For this review, take the finished solid that the model builds, in its own axes (mm). Give positions to 0.01 mm unless a question says otherwise; leave off trailing zeros. Write each loop counter-clockwise with the first axis right and the second up, starting at its lowest first coordinate (ties: lowest second). Pieces come first, ordered by that corner, then holes. Notation, with made-up numbers: M -5,23 L 17,23 A5 cw 17,31 Z; hole C -3.5,-29 d5. An arc over 180 degrees is marked long. One line per item, written item: value. Start each with the question number.
Item 1: Consider section B-B, the plane y = 1.2. Give the number of separate pieces and of enclosed holes in the cut face, and give its area (3 significant figures).
Item 2: Clearance check with flat-ended pins moving along their axes: pin 1 Ø3.5 at (x, z) = (70.83, -255.23) entering from +Y; pin 2 Ø10 at (x, z) = (48.5, -149) entering from -Y; pin 3 Ø1.6 at (y, z) = (1, -276) entering from -X (3 decimals). State where each tip first meets the part, or that it passes through.
Item 3: Consider section A-A, the plane z = -286. Write out the cut boundary in (x, y) (3 decimals), and give its area (3 significant figures).
Item 4: To check wall thickness, follow probe 1 along Z at (x, y) = (191.77, 0.9) (1 decimal); probe 2 along X at (y, z) = (1.3, 6.35); probe 3 along Z at (x, y) = (26, 0.2) (3 decimals). State the ranges of each line that lie inside material, in increasing order.
```python
from build123d import *

# Parameters (mm, degrees)
SKETCH1_W           = 210.82
SKETCH1_H           = 257.175
SKETCH1_W_2         = 185.42
SKETCH1_H_2         = 231.775
BOSS_EXTRUDE1_DEPTH = 3.175
SKETCH3_R           = 2.0955
CUT_EXTRUDE1_DEPTH  = 3.175
SKETCH3_3_R         = 45.33
SKETCH3_3_W         = 107.95
SKETCH3_3_H         = 21.4884
BOSS_EXTRUDE2_DEPTH = 3.175
FILLET1_R           = 2.54
SKETCH4_R           = 2.0955
CUT_EXTRUDE2_DEPTH  = 3.175


with BuildPart() as part:
    # Sketch1 → Boss-Extrude1 (new body)
    with BuildSketch(Plane(origin=(0, 0, 0), x_dir=(1, 0, 0), z_dir=(0, 1, 0))):
        with Locations((92.71, 115.8875)):
            Rectangle(SKETCH1_W, SKETCH1_H)
        with Locations((92.71, 115.8875)):
            Rectangle(SKETCH1_W_2, SKETCH1_H_2, mode=Mode.SUBTRACT)
        with Locations((92.71, 115.8875)):
            Rectangle(SKETCH1_W_2, SKETCH1_H_2)
    extrude(amount=BOSS_EXTRUDE1_DEPTH)

    # Sketch3 → Cut-Extrude1 (cut)
    with BuildSketch(Plane(origin=(0, 3.175, 0), x_dir=(1, 0, 0), z_dir=(0, 1, 0))):
        with Locations(Location((191.77, 238.125, 0), (0, 0, 270))):
            Circle(SKETCH3_R)
        with Locations(Location((191.77, -6.35, 0), (0, 0, 270))):
            Circle(SKETCH3_R)
        with Locations(Location((-6.35, -6.35, 0), (0, 0, 270))):
            Circle(SKETCH3_R)
        with Locations(Location((-6.35, 238.125, 0), (0, 0, 270))):
            Circle(SKETCH3_R)
    extrude(amount=-CUT_EXTRUDE1_DEPTH, mode=Mode.SUBTRACT)

    # Sketch3<3> → Boss-Extrude2 (add)
    with BuildSketch(Plane(origin=(0, 3.175, 0), x_dir=(1, 0, 0), z_dir=(0, 1, 0))):
        with BuildLine():
            ThreePointArc((138.04, 277.105), (134.430200877, 259.378360759), (124.175727387, 244.475))
            Line((124.175727387, 244.475), (146.685, 244.475))
            Line((146.685, 244.475), (146.685, 301.625))
            Line((146.685, 301.625), (142.4305, 301.625))
            ThreePointArc((142.4305, 301.625), (138.85325774, 300.14325774), (140.335, 303.7205))
            Line((140.335, 303.7205), (140.335, 307.975))
            Line((140.335, 307.975), (125.904156112, 307.975))
            ThreePointArc((125.904156112, 307.975), (134.897083311, 293.68989981), (138.04, 277.105))
        make_face()
        with BuildLine():
            Line((142.4305, 301.625), (146.685, 301.625))
            Line((146.685, 301.625), (146.685, 307.975))
            Line((146.685, 307.975), (140.335, 307.975))
            Line((140.335, 307.975), (140.335, 303.7205))
            ThreePointArc((140.335, 303.7205), (141.81674226, 303.10674226), (142.4305, 301.625))
        make_face()
        with BuildLine():
            Line((38.735, 244.475), (61.244272613, 244.475))
            ThreePointArc((61.244272613, 244.475), (47.396783015, 275.871603687), (59.515843888, 307.975))
            Line((59.515843888, 307.975), (45.085, 307.975))
            Line((45.085, 307.975), (45.085, 303.7205))
            ThreePointArc((45.085, 303.7205), (46.56674226, 303.10674226), (47.1805, 301.625))
            ThreePointArc((47.1805, 301.625), (45.085, 299.5295), (42.9895, 301.625))
            Line((42.9895, 301.625), (38.735, 301.625))
            Line((38.735, 301.625), (38.735, 244.475))
        make_face()
        with BuildLine():
            Line((38.735, 307.975), (38.735, 301.625))
            Line((38.735, 301.625), (42.9895, 301.625))
            ThreePointArc((42.9895, 301.625), (43.60325774, 303.10674226), (45.085, 303.7205))
            Line((45.085, 303.7205), (45.085, 307.975))
            Line((45.085, 307.975), (38.735, 307.975))
        make_face()
        with BuildLine():
            ThreePointArc((61.244272613, 244.475), (75.743989862, 235.069736233), (92.71, 231.775))
            Line((92.71, 231.775), (92.71, 244.475))
            Line((92.71, 244.475), (61.244272613, 244.475))
        make_face()
        with BuildLine():
            Line((92.71, 244.475), (92.71, 231.775))
            ThreePointArc((92.71, 231.775), (109.676010138, 235.069736233), (124.175727387, 244.475))
            Line((124.175727387, 244.475), (92.71, 244.475))
        make_face()
        with Locations((92.71, 277.105)):
            Circle(SKETCH3_3_R)
        with Locations((92.71, 318.7192)):
            Rectangle(SKETCH3_3_W, SKETCH3_3_H)
        with BuildLine():
            Line((59.515843888, 307.975), (92.71, 307.975))
            Line((92.71, 307.975), (92.71, 322.435))
            ThreePointArc((92.71, 322.435), (74.606522434, 318.663067809), (59.515843888, 307.975))
        make_face()
        with BuildLine():
            Line((92.71, 322.435), (92.71, 307.975))
            Line((92.71, 307.975), (125.904156112, 307.975))
            ThreePointArc((125.904156112, 307.975), (110.813477566, 318.663067809), (92.71, 322.435))
        make_face()
    extrude(amount=-BOSS_EXTRUDE2_DEPTH)

    # Fillet1
    fillet1_edges = [part.edges().sort_by_distance(p)[0] for p in [
        (146.685, 1.5875, -244.475),
        (38.735, 1.5875, -244.475),
        (38.735, 1.5875, -329.4634),
        (146.685, 1.5875, -329.4634),
        (-12.7, 1.5875, -244.475),
        (198.12, 1.5875, -244.475),
        (198.12, 1.5875, 12.7),
        (-12.7, 1.5875, 12.7),
    ]]
    fillet(fillet1_edges, radius=FILLET1_R)

    # Sketch4 → Cut-Extrude2 (cut)
    with BuildSketch(Plane(origin=(0, 3.175, 0), x_dir=(1, 0, 0), z_dir=(0, 1, 0))):
        with Locations(Location((70.834096089, 298.980903911, 0), (0, 0, 270))):
            Circle(SKETCH4_R)
        with Locations(Location((114.585903911, 298.980903911, 0), (0, 0, 270))):
            Circle(SKETCH4_R)
        with Locations(Location((114.585903911, 255.229096089, 0), (0, 0, 270))):
            Circle(SKETCH4_R)
        with Locations(Location((70.834096089, 255.229096089, 0), (0, 0, 270))):
            Circle(SKETCH4_R)
    extrude(amount=-CUT_EXTRUDE2_DEPTH, mode=Mode.SUBTRACT)


solid = part.part
```
Model answer:
1. separate pieces: 1
1. enclosed holes: 10
1. area: 63,200 mm2
2. pin 1: passes through
2. pin 2: stops at y = 0
2. pin 3: stops at x = 38.735
3. outline: M 38.735,0 L 146.685,0 L 146.685,3.175 L 38.735,3.175 Z
3. area: 343 mm2
4. probe 1: z = -244.5 to -240.2, -236 to 4.3, 8.4 to 12.7
4. probe 2: x = -12.7 to -8.45, -4.25 to 189.67, 193.87 to 198.12
4. probe 3: z = -244.475 to 12.7
